```python
from build123d import *

# Parameters (mm, degrees)
SKETCH1_W             = 12.7
SKETCH1_H             = 12.7
BOSS_EXTRUDE1_DEPTH   = 609.6
F_4_40_TAPPED_HOLE2_D = 2.2606


with BuildPart() as part:
    # Sketch1 → Boss-Extrude1 (new body)
    with BuildSketch(Plane(origin=(0, 0, 0), x_dir=(1, 0, 0), z_dir=(0, 1, 0))):
        Rectangle(SKETCH1_W, SKETCH1_H)
    extrude(amount=BOSS_EXTRUDE1_DEPTH)

    # Sketch8 → 1/4-20 Tapped Hole1 (revolve, cut)
    with BuildSketch(Plane(origin=(0, 0, 0), x_dir=(0, 0, -1), z_dir=(1, 0, 0))):
        Polygon((0, 0), (0, 14.233816902), (2.5527, 12.7), (2.5527, 0), align=None)
    f_1_4_20_tapped_hole1 = revolve(axis=Axis((0, -6.35, 0), (0, 1, 0)), mode=Mode.SUBTRACT)

    # #4-40 Tapped Hole2 (through all)
    with Locations(Plane(origin=(0, 17.752734497, 6.35), x_dir=(1, 0, 0), z_dir=(0, 0, 1))):
        with Locations((0, 0), (0, 247.65)):
            f_4_40_tapped_hole2 = Hole(F_4_40_TAPPED_HOLE2_D / 2)

    # Mirror1: 1/4-20 Tapped Hole1, #4-40 Tapped Hole2 across plane
    add(f_1_4_20_tapped_hole1.mirror(Plane.ZX.offset(304.8)), mode=Mode.SUBTRACT)
    add(f_4_40_tapped_hole2.mirror(Plane.ZX.offset(304.8)), mode=Mode.SUBTRACT)


solid = part.part
```
Work out the finished part from the listing and answer in its coordinate system (mm). Round coordinates to 2 decimals unless told otherwise and drop trailing zeros.
(1) The mould has two halves that part along X. Classify faces 1 (the flat face through (6.35, 301, 0)), 2 (the flat face through (-6.35, 301, 0)), 3 (the flat face through (3, 0, 0)): pulls with the +X half, pulls with the -X half, needs draft (parallel to the pull), parting line crosses it, or undercut.
Computed values:
face 1: pulls with the +X half
face 2: pulls with the -X half
face 3: needs draft
(2) This flat-tipped pin is pushed along its axis until it touches: P1, Ø4.5, axis at x = 0, z = 0, coming from the +Y side. Where does it stop, or does it pass through?
Computed values:
P1: stops at y = 596.72
(3) Find the intervals of material crossed by L1, parallel to Z at x = 0, y = 600.25; L2, parallel to Y at x = 0, z = -1.5; L3, parallel to Y at x = 0, z = 1, in increasing order.
Computed values:
L1: z = -6.35 to -2.55, 2.55 to 6.35
L2: y = 13.33 to 16.62, 18.88 to 264.27, 266.53 to 343.07, 345.33 to 590.72, 592.98 to 596.27
L3: y = 13.63 to 16.62, 18.88 to 264.27, 266.53 to 343.07, 345.33 to 590.72, 592.98 to 595.97
